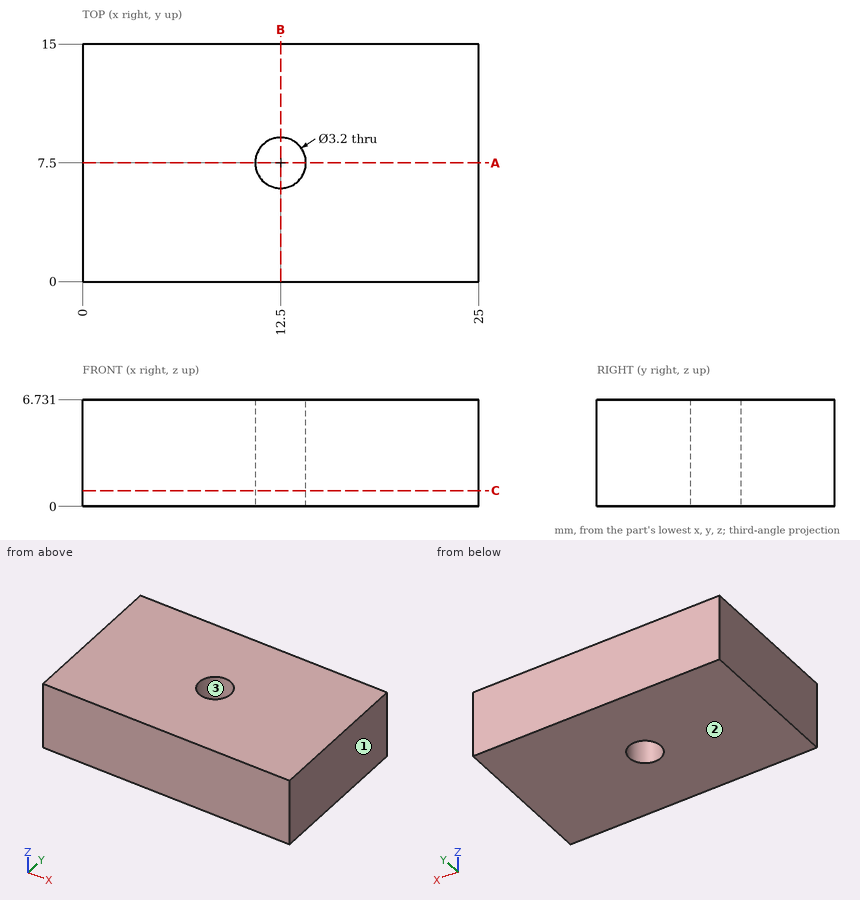
For this review, use the dimensioned drawing (mm, ordinates from the lowest corner) and the shaded views. Coordinates: 2 decimals unless noted, no trailing zeros. Loops run counter-clockwise (first coordinate to the right, second up) from the corner with the lowest first, then second, coordinate; pieces in that order, holes last. Notation, with made-up numbers: (-15, -14) - (16, -14) arc R23 cw to (16, 12) - close; hole circle Ø4 at (57, 80.25). An arc over 180 degrees is marked (long way). Use CSV: the item, a comma, the result in double quotes. Start each with the question number.
1) Consider section B-B on x = 12.5. Write out the cut boundary in (y, z).
2) Wall thickness on L1, parallel to Y at x = 12.5, z = 5.25; L2, parallel to X at y = 6.25, z = 5: over which ranges is each line inside the solid? List them lowest first. Write a range as from..to.
3) Consider section C-C on z = 1. Write out the cut boundary in (x, y).
4) The part is to be moulded in two halves that separate along X. For the marked faces 1, 2 and 3, say which applies: +X half, -X half, draft (parallel to the pull), parting line (faces both ways), or undercut.
5) Consider section A-A on y = 7.5. Write out the cut boundary in (x, z), then the cut area to 3 significant figures.
Geometry says:
1,outline,"(0, 0) - (5.9, 0) - (5.9, 6.73) - (0, 6.73) - close; (9.1, 0) - (15, 0) - (15, 6.73) - (9.1, 6.73) - close"
2,L1,"0..5.9, 9.1..15"
2,L2,"0..11.5, 13.5..25"
3,outline,"(0, 0) - (25, 0) - (25, 15) - (0, 15) - close; hole circle Ø3.2 at (12.5, 7.5)"
4,face 1,"+X half"
4,face 2,"draft"
4,face 3,"undercut"
5,outline,"(0, 0) - (10.9, 0) - (10.9, 6.73) - (0, 6.73) - close; (14.1, 0) - (25, 0) - (25, 6.73) - (14.1, 6.73) - close"
5,area,"147 mm^2"
